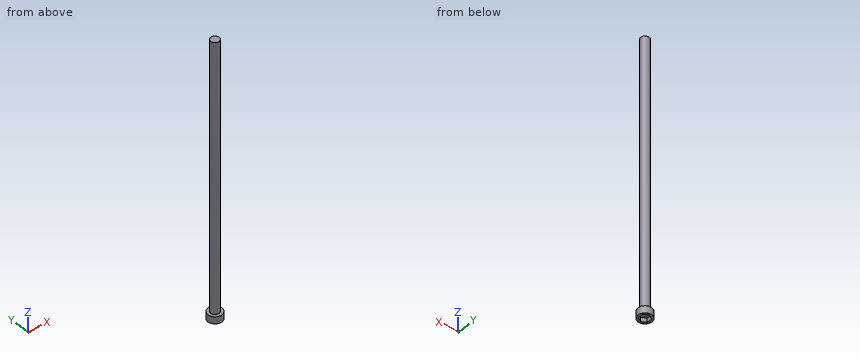
from build123d import *

# Parameters (mm, degrees)
SKETCH2_R           = 5
BOSS_EXTRUDE2_DEPTH = 5
CUT_EXTRUDE2_DEPTH  = 3
SKETCH6_R           = 3
BOSS_EXTRUDE3_DEPTH = 190


with BuildPart() as part:
    # Sketch2 → Boss-Extrude2 (new body)
    with BuildSketch(Plane.XY):
        Circle(SKETCH2_R)
    extrude(amount=BOSS_EXTRUDE2_DEPTH)

    # Sketch5 → Cut-Extrude2 (cut)
    with BuildSketch(Plane(origin=(0, 0, 0), x_dir=(-1, 0, 0), z_dir=(0, 0, -1))):
        Polygon((-3.229126368, 1.898971194), (-3.259120479, -1.847019869), (-0.029994111, -3.745991063), (3.229126368, -1.898971194), (3.259120479, 1.847019869), (0.029994111, 3.745991063), align=None)
    extrude(amount=-CUT_EXTRUDE2_DEPTH, mode=Mode.SUBTRACT)

    # Sketch6 → Boss-Extrude3 (add)
    with BuildSketch(Plane.XY.offset(5)):
        Circle(SKETCH6_R)
    extrude(amount=BOSS_EXTRUDE3_DEPTH)


solid = part.part
Here's how the part is built. I have some questions about the finished solid (model axes, mm). Give positions to 0.01 mm unless a question says otherwise; leave off trailing zeros. Order: outer loops, then holes, each group sorted by start corner. A loop starts at its lowest first (then second) coordinate and runs counter-clockwise, first axis right, second up. Notation, with made-up numbers: (87, 9) -> (125, 9) arc R7 cw to (125, 21) -> close; hole circle Ø8 at (-36.5, 36.25). An arc over 180 degrees is marked (long way). One line per item, written item: value. Start each with the question number.
1. Will these pins go through, and if not, where does the flat tip stop? pin 1 Ø6 at (y, z) = (1, 115.5) entering from +X; pin 2 Ø1.5 at (x, z) = (1, 97) entering from -Y; pin 3 Ø6 at (x, z) = (-2.5, 92) entering from +Y.
2. I need wall thicknesses on probe 1 along X at (y, z) = (0.25, 113); probe 2 along Z at (x, y) = (-0.5, -1.5); probe 3 along Z at (x, y) = (-2.75, 4). Which ranges of each line are inside material? Lowest first, please. Write a range as from..to.
3. Imagine slicing it at A-A, the plane z = 26. List the corners of the cut face in (x, y) for me, plus the area to 3 significant figures.
Values follow:
1. pin 1: stops at x = 3
1. pin 2: stops at y = -2.99
1. pin 3: stops at y = 3
2. probe 1: x = -2.99..2.99
2. probe 2: z = 3..195
2. probe 3: z = 0..5
3. outline: circle Ø6 at (0, 0)
3. area: 28.3 mm2
